Autodesk Inventor part; units mm, degrees
ref_plane "YZ Plane" through (0, 0, 0) normal (1, 0, 0) x (0, 1, 0)
ref_plane "XZ Plane" through (0, 0, 0) normal (0, 1, 0) x (-1, 0, 0)
ref_plane "XY Plane" through (0, 0, 0) normal (0, 0, 1) x (1, 0, 0)
sketch "Sketch1" plane through (0, 0, 0) normal (0, 1, 0) x (-1, 0, 0)
  line L0 (0, -3) -> (-10, -3)
  circle A0 centre (-21.6, 10.775) radius 1.5
  line L1 (0, 35) -> (-45, 35)
  line L2 (0, 0) -> (0, 35)
  circle A1 centre (-29.1, -16.775) radius 1.5
  arc A2 (-17.7405, 9.7243) -> (-25.4595, 11.8257) centre (-21.6, 10.775) ccw
  arc A3 (-32.9595, -15.7243) -> (-25.2405, -17.8257) centre (-29.1, -16.775) ccw
  line L3 (-17.7405, 9.7243) -> (-25.2405, -17.8257)
  line L4 (-27.4538, 4.5) -> (-35.4538, 4.5)
  line L5 (-35.4538, 4.5) -> (-35.4538, -10.5)
  line L6 (-35.4538, -10.5) -> (-31.5373, -10.5)
  line L7 (-25.4595, 11.8257) -> (-27.4538, 4.5)
  line L8 (-31.5373, -10.5) -> (-32.9595, -15.7243)
  point P0 (-35.4538, -3)
  dimension "d0" = 10
  dimension "d1" = 3
  dimension "d2" = 13.775
  dimension "d3" = 3
  dimension "d7" = 45
  dimension "d8" = 35
  dimension "d9" = 23.4
  dimension "d10" = 3
  dimension "d11" = 13.775
  dimension "d12" = 15.9
  dimension "d13" = 2.5
  dimension "d14" = 2.5
  dimension "d15" = 15
  dimension "d16" = 8
extrude "Extrusion1" add sketch "Sketch1" along normal blind 2.7
fillet "Fillet1" radius 2 4 edges at (35.4538, 1.35, 4.5) (27.4538, 1.35, 4.5) (35.4538, 1.35, -10.5) (31.5373, 1.35, -10.5)
properties part number "SujecionServo"
Can you work these out from the model? Positions are in its coordinate system, mm. A direction names the side the tool comes from. Round coordinates to 2 decimals unless told otherwise and drop trailing zeros. Loops run counter-clockwise (first coordinate to the right, second up) from the corner with the lowest first, then second, coordinate; pieces in that order, holes last.
Item 1: Suppose I cut it at C-C, the plane z = 5.5. Write out the boundary of the cut face in (x, y).
Item 2: Suppose I cut it at D-D, the plane y = 1.45. State how many separate pieces and enclosed holes the cut face has, then the cut area to 3 significant figures.
Item 3: Which directions (+Z, -Z, +X, -X, +Y, -Y) give clear straight access to the entire face, cutting with the end or side of a thin tool? Please do faces 1 (the flat face through (32.58, 1.33, -14.33)), 2 (the flat face through (35.454, 1, -3)).
Item 4: Please list where these lines run through material, in increasing order: L1, parallel to X at y = 2.5, z = -18; L2, parallel to X at y = 2.2, z = 9; L3, parallel to Z at x = 29.5, y = 1.2.
Item 5: Will these pins go through, and if not, where does the flat tip stop? pin 1 Ø1 at (y, z) = (1, -1) entering from -X; pin 2 Ø1.4 at (x, y) = (32, 2) entering from +Z.
Item 6: Suppose I cut it at B-B, the plane x = 28. Write out the boundary of the cut face in (y, z), then the cut area to 3 significant figures.
Item 7: Suppose I cut it at A-A, the plane x = 21.6. Write out the boundary of the cut face in (y, z) (3 decimals).
Item 8: If we mould it in two halves opening along Z, with no side actions, what happens to faces 3 (the cylindrical face through (27.67, 1.33, -17.23)), 4 (the flat face through (21.44, 1.33, -3.86)), 5 (the flat face through (31, 1, 4.5))? For each: +Z half, -Z half, draft (parallel to the pull), parting line (faces both ways), or undercut.
Reported:
1. outline: (18.89, 0) - (27.25, 0) - (27.25, 2.7) - (18.89, 2.7) - close
2. separate pieces: 1
2. enclosed holes: 2
2. area: 354 mm2
3. face 1: +X, +Y, -Y
3. face 2: +Z, -Z, +X, +Y, -Y
4. L1: x = 25.29 to 28.23, 29.97 to 32.91
4. L2: x = 17.94 to 26.23
4. L3: z = -20.75 to -18.22, -15.33 to 4.5
5. pin 1: stops at x = 20.52
5. pin 2: stops at z = 4.5
6. outline: (0, -20.62) - (2.7, -20.62) - (2.7, -17.79) - (0, -17.79) - close; (0, -15.76) - (2.7, -15.76) - (2.7, 4.76) - (0, 4.76) - close
6. area: 63.0 mm2
7. outline: (0, -4.453) - (2.7, -4.453) - (2.7, 9.275) - (0, 9.275) - close; (0, 12.275) - (2.7, 12.275) - (2.7, 14.775) - (0, 14.775) - close
8. face 3: undercut
8. face 4: -Z half
8. face 5: +Z half
